Could you check a few things on this model? Use its own coordinates, in mm. Face numbers are marked on the shaded views. A direction names the side the tool comes from. Round coordinates to 2 decimals unless told otherwise and drop trailing zeros. Write each loop counter-clockwise with the first axis right and the second up, starting at its lowest first coordinate (ties: lowest second). Pieces come first, ordered by that corner, then holes. Notation, with made-up numbers: (84, -35.5) - (142, -35.5) arc R28 ccw to (142, -8.5) - close; hole circle Ø10 at (-34.5, 31). An arc over 180 degrees is marked (long way). Write each question's results on one line, items separated by ' | '. Start each with the question number.
(1) Imagine slicing it at B-B on z = -65.5. Write out the boundary of the cut face in (x, y) (3 decimals).
(2) Imagine slicing it at A-A on z = -25.4. Write out the boundary of the cut face in (x, y) (3 decimals).
(3) Thinking about a two-plate mould opening in Y: for the marked faces 3, 4 and 5, which applies, +Y half, -Y half, draft (parallel to the pull), parting line (faces both ways), or undercut?
(4) Imagine slicing it at C-C on y = 8.5. Write out the boundary of the cut face in (x, z) (3 decimals), then the cut area to 3 significant figures.
(5) On a 3-axis mill with a long thin cutter (end or side, diameter ignored), from which of +Z, -Z, +X, -X, +Y, -Y can I reach the whole of each face in a straight line? I mean the marked faces 1 and 2. Say none if no direction works.
(6) Please list where these lines run through material, in increasing order: line 1 (Y direction, x = 17.25, z = -193.5) (3 decimals); line 2 (X direction, y = 47, z = -26) (3 decimals); line 3 (Y direction, x = 1, z = -154.5). Write a range as [from, to].
(7) For P1, Ø3, axis at x = 13.843, z = -203.2, coming from the +Y side; P2, Ø12, axis at y = 43.5, z = -119.5, coming from the +X side, each with a flat end and sliding along its axis, tell me the tip position at first contact or that it passes through.
```python
from build123d import *

# Parameters (mm, degrees)
SKETCH1_W                      = 228.6
SKETCH1_H                      = 63.5
BASE_FLANGE1_DEPTH             = 3.175
EDGE_FLANGE1_STRIP_W           = 19.05
EDGE_FLANGE1_STRIP_H           = 3.175
EDGE_FLANGE1_STRIP_CUT_DEPTH   = 228.6
EDGE_FLANGE1_STRIP_2_W         = 19.05
EDGE_FLANGE1_STRIP_2_H         = 3.175
EDGE_FLANGE1_STRIP_CUT_2_DEPTH = 228.6
EDGE_FLANGE1_DEPTH             = 228.6
EDGE_FLANGE1_BEND_DEPTH        = 228.6
SKETCH12_R                     = 2.45745
CUT_EXTRUDE1_DEPTH             = 239.403593564
FILLET1_R                      = 3.175


# Sheet-metal steps are written as plain solids
with BuildPart() as part:
    # Sketch1 → Base-Flange1 (new body)
    with BuildSketch(Plane(origin=(0, 0, 0), x_dir=(0, 0, -1), z_dir=(1, 0, 0))):
        with Locations((114.3, 31.75)):
            Rectangle(SKETCH1_W, SKETCH1_H)
    extrude(amount=-BASE_FLANGE1_DEPTH)

    # Edge-Flange1 strip (across the edge) → Edge-Flange1 strip cut (cut)
    with BuildSketch(Plane(origin=(0, 63.5, -228.6), x_dir=(0, -1, 0), z_dir=(0, 0, 1))):
        with Locations((-3.175, -1.5875)):
            Rectangle(EDGE_FLANGE1_STRIP_W, EDGE_FLANGE1_STRIP_H)
    extrude(amount=EDGE_FLANGE1_STRIP_CUT_DEPTH, mode=Mode.SUBTRACT)

    # Edge-Flange1 strip 2 (across the edge) → Edge-Flange1 strip cut 2 (cut)
    with BuildSketch(Plane.YX):
        with Locations((-3.175, -1.5875)):
            Rectangle(EDGE_FLANGE1_STRIP_2_W, EDGE_FLANGE1_STRIP_2_H)
    extrude(amount=EDGE_FLANGE1_STRIP_CUT_2_DEPTH, mode=Mode.SUBTRACT)

    # Edge-Flange1 section (across the edge) → Edge-Flange1 (add)
    with BuildSketch(Plane(origin=(0, 63.5, -228.6), x_dir=(0, -1, 0), z_dir=(0, 0, 1))):
        with BuildLine():
            Line((0, 3.175), (0, 23.368))
            Line((0, 23.368), (3.175, 23.368))
            Line((3.175, 23.368), (3.175, 3.175))
            ThreePointArc((3.175, 3.175), (4.10493597, 0.92993597), (6.35, 0))
            Line((6.35, 0), (6.35, -3.175))
            ThreePointArc((6.35, -3.175), (1.859871939, -1.315128061), (0, 3.175))
        make_face()
    extrude(amount=EDGE_FLANGE1_DEPTH)

    # Edge-Flange1 section 2 (across the edge) → Edge-Flange1 bend (add)
    with BuildSketch(Plane.YX):
        with BuildLine():
            Line((0, 3.175), (0, 23.368))
            Line((0, 23.368), (3.175, 23.368))
            Line((3.175, 23.368), (3.175, 3.175))
            ThreePointArc((3.175, 3.175), (4.10493597, 0.92993597), (6.35, 0))
            Line((6.35, 0), (6.35, -3.175))
            ThreePointArc((6.35, -3.175), (1.859871939, -1.315128061), (0, 3.175))
        make_face()
    extrude(amount=EDGE_FLANGE1_BEND_DEPTH)

    # Sketch12 → Cut-Extrude1 (cut, through all)
    with BuildSketch(Plane(origin=(0, 63.5, 0), x_dir=(1, 0, 0), z_dir=(0, 1, 0))):
        with Locations(Location((13.843, 203.2, 0), (0, 0, 180))):
            Circle(SKETCH12_R)
        with Locations(Location((13.843, 25.4, 0), (0, 0, 180))):
            Circle(SKETCH12_R)
    extrude(amount=-CUT_EXTRUDE1_DEPTH, mode=Mode.SUBTRACT)

    # Fillet1
    fillet1_edges = [part.edges().sort_by_distance(p)[0] for p in [
        (23.368, 61.9125, -228.6),
        (23.368, 61.9125, 0),
        (23.368, 1.5875, 0),
        (23.368, 1.5875, -228.6),
    ]]
    fillet(fillet1_edges, radius=FILLET1_R)


solid = part.part
```
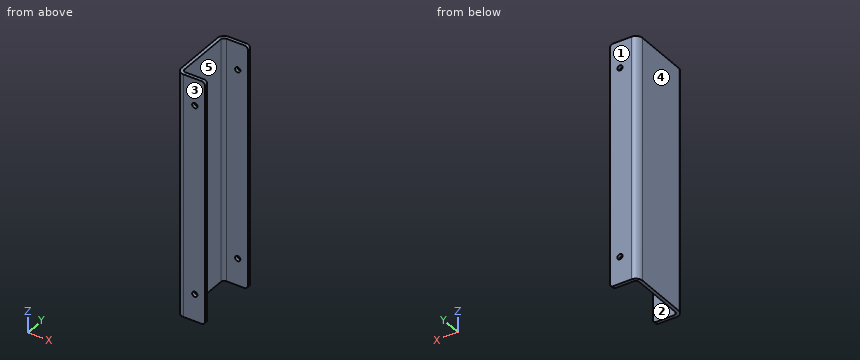
Response:
1) outline: (-3.175, 6.35) arc R6.35 ccw to (3.175, 0) - (23.368, 0) - (23.368, 3.175) - (3.175, 3.175) arc R3.175 cw to (0, 6.35) - (0, 57.15) arc R3.175 cw to (3.175, 60.325) - (23.368, 60.325) - (23.368, 63.5) - (3.175, 63.5) arc R6.35 ccw to (-3.175, 57.15) - close
2) outline: (-3.175, 6.35) arc R6.35 ccw to (3.175, 0) - (11.386, 0) - (11.386, 3.175) - (3.175, 3.175) arc R3.175 cw to (0, 6.35) - (0, 57.15) arc R3.175 cw to (3.175, 60.325) - (11.386, 60.325) - (11.386, 63.5) - (3.175, 63.5) arc R6.35 ccw to (-3.175, 57.15) - close; (16.3, 0) - (23.368, 0) - (23.368, 3.175) - (16.3, 3.175) - close; (16.3, 60.325) - (23.368, 60.325) - (23.368, 63.5) - (16.3, 63.5) - close
3) face 3: -Y half | face 4: draft | face 5: undercut
4) outline: (-3.175, -228.6) - (0, -228.6) - (0, 0) - (-3.175, 0) - close | area: 726 mm²
5) face 1: +Z, -Z, +X, -X, +Y | face 2: +Z, -Z, +X
6) line 1: [0, 3.175], [60.325, 63.5] | line 2: [-3.175, 0] | line 3: [0.38, 4.04], [59.46, 63.12]
7) P1: through | P2: x = 0
